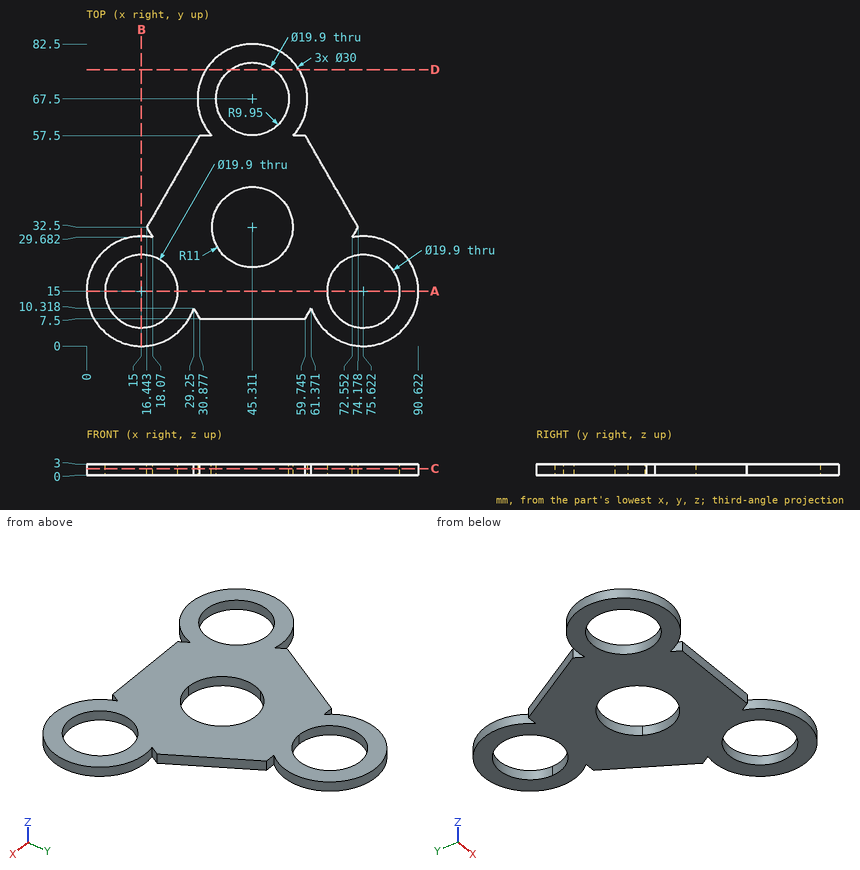
Print and shaded views of the part. All mm, measured from the part's lowest x, y and z. Round coordinates to 2 decimals unless told otherwise and drop trailing zeros. Write each loop counter-clockwise with the first axis right and the second up, starting at its lowest first coordinate (ties: lowest second). Pieces come first, ordered by that corner, then holes. Notation, with made-up numbers: M 8.25,23.25 L 58.25,23.25 A3 cw 58.25,28.25 Z; hole C 2,31.5 d7. An arc over 180 degrees is marked long. Use a Markdown table: item, result. Add a question column.
1. Drill centre lines: probe 1 along Y at (x, z) = (46, 0.95) (1 decimal); probe 2 along Y at (x, z) = (36.5, 0.25) (1 decimal); probe 3 along X at (y, z) = (14.5, 2.2) (1 decimal). Where is each one in solid material? Low to high.
2. Slice it at D-D on y = 75.5. Give the cut face in (x, z) (1 decimal).
3. Slice it at A-A on y = 15. Give the cut face in (x, z).
4. Slice it at B-B on x = 15. Give the cut face in (y, z), then the cut area to 3 significant figures.
5. Flat gauge pins, fed straight in: P1, Ø8, axis at x = 49, y = 27.5, coming from the +Z side; P2, Ø23, axis at x = 15, y = 15, coming from the -Z side; P3, Ø1, axis at x = 76.5, z = 2, coming from the -Y side (1 decimal); P4, Ø0.9, axis at x = 48, z = 1.5, coming from the -Y side. Where does each tip first touch, or does it go through?
6. Slice it at C-C on z = 1.8. Give the number of separate pieces and of enclosed holes in the cut face, then the cut area to 3 significant figures.
Reply:
| question | item | result |
|---|---|---|
| 1 | probe 1 | y = 7.5 to 21.5, 43.5 to 57.6, 77.4 to 82.5 |
| 1 | probe 2 | y = 7.5 to 25.9, 39.1 to 62.9, 72.1 to 79.6 |
| 1 | probe 3 | x = 0 to 5.1, 24.9 to 65.7, 85.6 to 90.6 |
| 2 | outline | M 32.6,0 L 39.4,0 L 39.4,3 L 32.6,3 Z; M 51.2,0 L 58,0 L 58,3 L 51.2,3 Z |
| 3 | outline | M 0,0 L 5.05,0 L 5.05,3 L 0,3 Z; M 24.95,0 L 65.67,0 L 65.67,3 L 24.95,3 Z; M 85.57,0 L 90.62,0 L 90.62,3 L 85.57,3 Z |
| 4 | outline | M 0,0 L 5.05,0 L 5.05,3 L 0,3 Z; M 24.95,0 L 30,0 L 30,3 L 24.95,3 Z |
| 4 | area | 30.3 mm^2 |
| 5 | P1 | passes through |
| 5 | P2 | stops at z = 0 |
| 5 | P3 | stops at y = 0 |
| 5 | P4 | stops at y = 7.5 |
| 6 | separate pieces | 1 |
| 6 | enclosed holes | 4 |
| 6 | area | 2,740 mm^2 |
